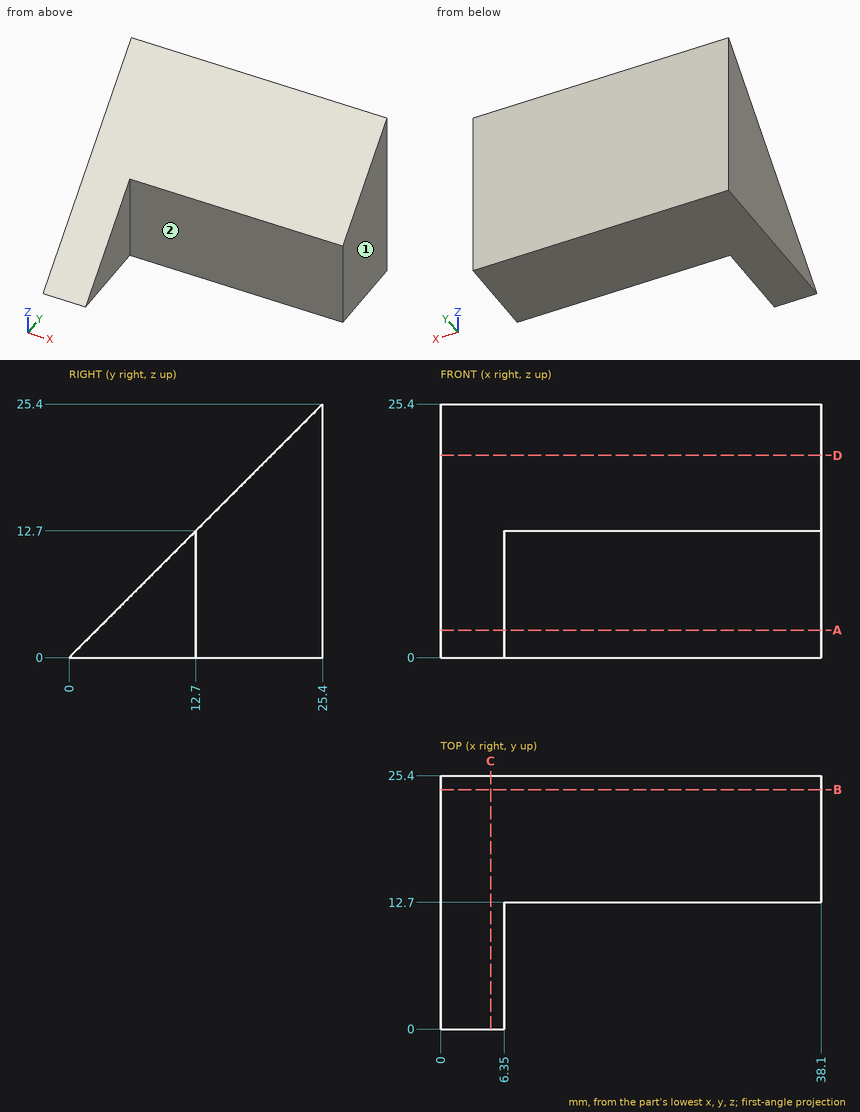
Part print with two shaded views. Sizes in mm from the minimum x, y, z corner. A direction names the side the tool comes from. Round coordinates to 2 decimals unless told otherwise and drop trailing zeros. Loops run counter-clockwise (first coordinate to the right, second up) from the corner with the lowest first, then second, coordinate; pieces in that order, holes last. Notation, with made-up numbers: (-37, 31) - (-9, 31) arc R20 ccw to (-9, 43) - close; hole circle Ø11 at (25, 36). An arc over 180 degrees is marked (long way). Put each result on its own line as item: value.
1. 3-axis set-ups, long thin cutter, end or side, ignore diameter. For the marked faces 1 and 2: which of +Z, -Z, +X, -X, +Y, -Y reach the whole face in a straight line?
Geometry check:
face 1: +Z, -Z, +X, +Y, -Y
face 2: +Z, -Z, +X, -Y
2. Wall check: line 1 (Y direction, x = 35, z = 4.25); line 2 (X direction, y = 9.5, z = 5.5); line 3 (Z direction, x = 2.5, y = 13). Give the ranges that are in metal, low to high.
Geometry check:
line 1: 12.7 to 25.4
line 2: 0 to 6.35
line 3: 0 to 13
3. Pin check, flat tips, straight feed: P1, Ø2, axis at x = 29.5, y = 21, coming from the +Z side; P2, Ø5, axis at x = 33.5, z = 14.5, coming from the -Y side; P3, Ø10, axis at x = 31.5, y = 13, coming from the +Z side. Stop position of each tip, or through.
Geometry check:
P1: z = 22
P2: y = 12.7
P3: z = 18
4. Slice it at A-A on z = 2.75. List the corners of the cut face in (x, y).
Geometry check:
outline: (0, 2.75) - (6.35, 2.75) - (6.35, 12.7) - (38.1, 12.7) - (38.1, 25.4) - (0, 25.4) - close
5. Slice it at B-B on y = 24. List the corners of the cut face in (x, z).
Geometry check:
outline: (0, 0) - (38.1, 0) - (38.1, 24) - (0, 24) - close
6. Slice it at C-C on x = 5. List the corners of the cut face in (y, z).
Geometry check:
outline: (0, 0) - (25.4, 0) - (25.4, 25.4) - close
7. Slice it at D-D on z = 20.25. List the corners of the cut face in (x, y), and give its area (3 significant figures).
Geometry check:
outline: (0, 20.25) - (38.1, 20.25) - (38.1, 25.4) - (0, 25.4) - close
area: 196 mm²
